For this review, take the finished solid that the model builds, in its own axes (mm). Give positions to 0.01 mm unless a question says otherwise; leave off trailing zeros. Order: outer loops, then holes, each group sorted by start corner. A loop starts at its lowest first (then second) coordinate and runs counter-clockwise, first axis right, second up. Notation, with made-up numbers: (77.5, 39) - (136.5, 39) arc R25 ccw to (136.5, 74) - close; hole circle Ø11 at (71, 65). An arc over 180 degrees is marked (long way). One line per item, written item: value.
```python
from build123d import *

# Parameters (mm, degrees)
SKETCH_1_W          = 120
SKETCH_1_H          = 29
EXTRUDE_1_DEPTH     = 3
SKETCH_2_W          = 76
SKETCH_2_H          = 3.5
CUT_EXTRUDE_1_DEPTH = 62.800080906
SKETCH_3_R          = 0.35
CUT_EXTRUDE_2_DEPTH = 3
SKETCH_5_R          = 0.35
CUT_EXTRUDE_3_DEPTH = 3


with BuildPart() as part:
    # 草图1 → 凸台-拉伸1 (new body)
    with BuildSketch(Plane(origin=(0, 0, 0), x_dir=(1, 0, 0), z_dir=(0, 1, 0))):
        Rectangle(SKETCH_1_W, SKETCH_1_H)
    extrude(amount=EXTRUDE_1_DEPTH)

    # 草图2 → 切除-拉伸1 (cut, through all)
    with BuildSketch(Plane.XZ):
        with Locations((22, -12.75)):
            Rectangle(SKETCH_2_W, SKETCH_2_H)
    extrude(amount=-CUT_EXTRUDE_1_DEPTH, mode=Mode.SUBTRACT)

    # 草图3 → 切除-拉伸2 (cut)
    with BuildSketch(Plane(origin=(60, 0, 0), x_dir=(0, 0, -1), z_dir=(1, 0, 0))):
        with Locations((-8.125, 1.5)):
            Circle(SKETCH_3_R)
        with Locations((4.625, 1.5)):
            Circle(SKETCH_3_R)
    extrude(amount=-CUT_EXTRUDE_2_DEPTH, mode=Mode.SUBTRACT)

    # 草图5 → 切除-拉伸3 (cut)
    with BuildSketch(Plane.XY.offset(14.5)):
        with Locations((-29.25, 1.5)):
            Circle(SKETCH_5_R)
        with Locations((1.5, 1.5)):
            Circle(SKETCH_5_R)
        with Locations((32.25, 1.5)):
            Circle(SKETCH_5_R)
    extrude(amount=-CUT_EXTRUDE_3_DEPTH, mode=Mode.SUBTRACT)


solid = part.part
```
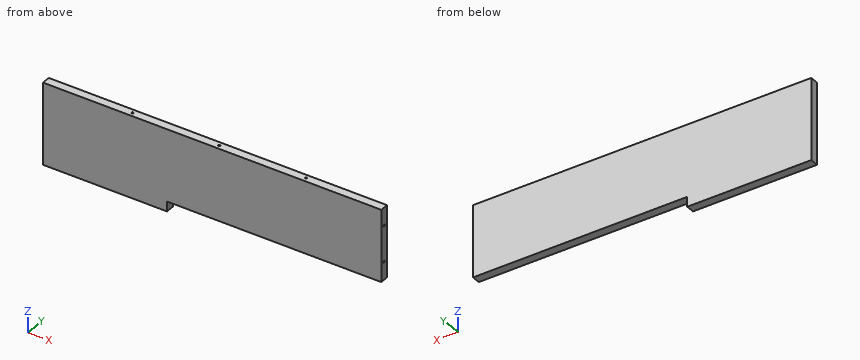
(1) Take a section at A-A (y = 0.6). Write out the cut boundary in (x, z), then the cut area to 3 significant figures.
Answers below:
outline: (-60, -14.5) - (-16, -14.5) - (-16, -11) - (60, -11) - (60, 14.5) - (-60, 14.5) - close
area: 3,210 mm^2
(2) Take a section at C-C (z = -12.5). Write out the cut boundary in (x, y).
Answers below:
outline: (-60, 0) - (-16, 0) - (-16, 3) - (-60, 3) - close
(3) For P1, Ø0.9, axis at y = 1.5, z = -13, coming from the +X side; P2, Ø0.6, axis at x = 1.5, y = 1.5, coming from the +Z side, all flat-tipped, find the tip position at first contact; note any pin that passes through.
Answers below:
P1: stops at x = -16
P2: stops at z = 11.5
(4) Wall thickness on line 1 (Y direction, x = 32.25, z = 13.6); line 2 (Z direction, x = 22, y = 2.85); line 3 (X direction, y = 1.4, z = 8): over which ranges is each line inside the solid? List them lowest first. Write a range as from..to.
Answers below:
line 1: y = 0..1.15, 1.85..3
line 2: z = -11..14.5
line 3: x = -60..57
(5) Take a section at B-B (x = 40.5). Write out the cut boundary in (y, z).
Answers below:
outline: (0, -11) - (3, -11) - (3, 14.5) - (0, 14.5) - close
